```python
from build123d import *

# Parameters (mm, degrees)
PAD005_DEPTH           = 100
PAD005_DEPTH_BACK      = 10
PAD004_DEPTH           = 60
PAD004_DEPTH_BACK      = 10
BOX_W                  = 55.2
BOX_H                  = 91.2
BOX_DEPTH              = 5.5
BOX_PLACEMENT_ANGLE    = -90
BOX001_W               = 56.2
BOX001_H               = 92.2
BOX001_DEPTH           = 1
BOX001_PLACEMENT_ANGLE = -90


with BuildPart() as pad_bezel_top_bottom:
    # Sketch006 → Pad005 (new body, two sides)
    with BuildSketch(Plane.YZ) as pad005_sk:
        Polygon((3.1, -1), (-0.4, -1), (-0.4, -0.6), (0, -0.6), (2.1, 4.5), (2.6, 4.5), (2.6, 0), (3.1, 0), align=None)
        Polygon((-51.5, -0.6), (-52.099998, 4.5), (-52.599998, 4.5), (-52.599998, 0), (-53.1, 0), (-53.1, -1), (-51.1, -1), (-51.1, -0.6), align=None)
    extrude(amount=PAD005_DEPTH)
    extrude(pad005_sk.sketch, amount=-PAD005_DEPTH_BACK)


with BuildPart() as fusion:
    # Sketch005 → Pad004 (new body, two sides)
    with BuildSketch(Plane.XZ) as pad004_sk:
        Polygon((-3.1, -1), (0.4, -1), (0.4, -0.6), (0, -0.6), (-2.1, 4.5), (-2.6, 4.5), (-2.6, 0), (-3.1, 0), align=None)
        Polygon((85.6, -1), (89.1, -1), (89.1, 0), (88.6, 0), (88.6, 4.5), (88.1, 4.5), (86, -0.6), (85.6, -0.6), align=None)
    extrude(amount=PAD004_DEPTH)
    extrude(pad004_sk.sketch, amount=-PAD004_DEPTH_BACK)

    # Fusion: union Pad (bezel top/bottom)
    add(pad_bezel_top_bottom.part)


with BuildPart() as cube_bezel_main:
    # Box → Box (new body)
    with BuildSketch(Plane.XY):
        with Locations((27.6, 45.6)):
            Rectangle(BOX_W, BOX_H)
    extrude(amount=BOX_DEPTH)


with BuildPart() as cube_bezel_main_1:
    # Box placement: moved
    add(cube_bezel_main.part.moved(Location((-2.6, 2.6, 0))).rotate(Axis((-2.6, 2.6, 0), (0, 0, 1)), BOX_PLACEMENT_ANGLE))


with BuildPart() as common_bezel:
    # Box001 → Box001 (new body)
    with BuildSketch(Plane.XY):
        with Locations((28.1, 46.1)):
            Rectangle(BOX001_W, BOX001_H)
    extrude(amount=BOX001_DEPTH)


with BuildPart() as common_bezel_1:
    # Box001 placement: moved
    add(common_bezel.part.moved(Location((-3.1, 3.1, -1))).rotate(Axis((-3.1, 3.1, -1), (0, 0, 1)), BOX001_PLACEMENT_ANGLE))

    # Fusion001: union Cube (bezel main)
    add(cube_bezel_main_1.part)

    # Common: intersect Fusion
    add(fusion.part, mode=Mode.INTERSECT)


solid = common_bezel_1.part
```
Source: CAD feature listing. Evaluate the final solid. Frame: model axes, mm. A direction names the side the tool comes from. Coordinates: 2 decimals unless noted, no trailing zeros. Write each loop counter-clockwise with the first axis right and the second up, starting at its lowest first coordinate (ties: lowest second). Pieces come first, ordered by that corner, then holes. Notation, with made-up numbers: (-8, 30) -> (34, 30) arc R17 cw to (34, 36) -> close; hole circle Ø2 at (72.5, -22). An arc over 180 degrees is marked (long way). Return JSON: item names as keys, results as strings. Group by question number.
1) Ray query, line 1 along Y through (x, z) = (50, 3.35); line 2 along X through (y, z) = (-47.5, 3.2); line 3 along Y through (x, z) = (55.5, 2.1). Return the intervals inside material, ascending.
2) Set-up query: faces 1 (the face through (-2, -52.6, 2)), 2 (the face through (-2.6, -25, 2)), 3 (the face through (42, 2.6, 2)), 4 (the face through (43.631, -51.796, 1.914)). Return all of +Z, -Z, +X, -X, +Y, -Y with unobstructed straight access to the full face (end or side cutting, diameter ignored); none if empty.
3) Section query C-C, the plane x = 13. Return loops of the section in (y, z).
4) Contact query for flat-ended pins moving along their axis: P1, Ø1.3, axis at y = -35, z = 2, coming from the -X side; P2, Ø1.3, axis at y = -12.5, z = 2.5, coming from the +X side; P3, Ø1.4, axis at x = 58, z = 1, coming from the -Y side. Output: stop coordinate, or through.
5) Section query A-A, the plane y = -50. Return loops of the section in (x, z).
From the geometry:
{
 "1": {"line 1": "-52.6 to -51.96, 1.63 to 2.6", "line 2": "-2.6 to -1.56, 87.56 to 88.6", "line 3": "-52.6 to -51.82, 1.11 to 2.6"},
 "2": {"face 1": "+Z, +X, -X, -Y", "face 2": "+Z, -X, +Y, -Y", "face 3": "+Z, +X, -X, +Y", "face 4": "+Z"},
 "3": {"outline": "(-53.1, -1) -> (-51.1, -1) -> (-51.1, -0.6) -> (-51.5, -0.6) -> (-52.1, 4.5) -> (-52.6, 4.5) -> (-52.6, 0) -> (-53.1, 0) -> close; (-0.4, -1) -> (3.1, -1) -> (3.1, 0) -> (2.6, 0) -> (2.6, 4.5) -> (2.1, 4.5) -> (0, -0.6) -> (-0.4, -0.6) -> close"},
 "4": {"P1": "x = -2.6", "P2": "x = 88.6", "P3": "y = -52.6"},
 "5": {"outline": "(-3.1, -1) -> (0.4, -1) -> (0.4, -0.6) -> (0, -0.6) -> (-2.1, 4.5) -> (-2.6, 4.5) -> (-2.6, 0) -> (-3.1, 0) -> close; (85.6, -1) -> (89.1, -1) -> (89.1, 0) -> (88.6, 0) -> (88.6, 4.5) -> (88.1, 4.5) -> (86, -0.6) -> (85.6, -0.6) -> close"}
}
